from build123d import *

# Parameters (mm, degrees)
DODANIE_WYCI_GNI_CIE1_DEPTH = 15
SZKIC1_3_R                  = 6
DODANIE_WYCI_GNI_CIE2_DEPTH = 1
SZKIC1_4_R                  = 6
SZKIC1_4_R_2                = 5
DODANIE_WYCI_GNI_CIE3_DEPTH = 11
ZAOKR_GLENIE1_R             = 3
ZAOKR_GLENIE2_R             = 0.5
ZAOKR_GLENIE3_R             = 1


with BuildPart() as part:
    # Szkic1 → Dodanie-wyci_gni_cie1 (new body)
    with BuildSketch(Plane(origin=(0, 0, 0), x_dir=(1, 0, 0), z_dir=(0, 1, 0))):
        with BuildLine():
            Line((-26.353622573, 20), (26.353622573, 20))
            ThreePointArc((26.353622573, 20), (32.113981294, 17.613981294), (34.5, 11.853622573))
            Line((34.5, 11.853622573), (34.5, -11.853622573))
            ThreePointArc((34.5, -11.853622573), (32.113981294, -17.613981294), (26.353622573, -20))
            Line((26.353622573, -20), (-26.353622573, -20))
            ThreePointArc((-26.353622573, -20), (-32.113981294, -17.613981294), (-34.5, -11.853622573))
            Line((-34.5, -11.853622573), (-34.5, 11.853622573))
            ThreePointArc((-34.5, 11.853622573), (-32.113981294, 17.613981294), (-26.353622573, 20))
        make_face()
        with BuildLine():
            Line((-26.353622573, 19), (26.353622573, 19))
            ThreePointArc((26.353622573, 19), (31.406874513, 16.906874513), (33.5, 11.853622573))
            Line((33.5, 11.853622573), (33.5, -11.853622573))
            ThreePointArc((33.5, -11.853622573), (31.406874513, -16.906874513), (26.353622573, -19))
            Line((26.353622573, -19), (-26.353622573, -19))
            ThreePointArc((-26.353622573, -19), (-31.406874513, -16.906874513), (-33.5, -11.853622573))
            Line((-33.5, -11.853622573), (-33.5, 11.853622573))
            ThreePointArc((-33.5, 11.853622573), (-31.406874513, 16.906874513), (-26.353622573, 19))
        make_face(mode=Mode.SUBTRACT)
    extrude(amount=DODANIE_WYCI_GNI_CIE1_DEPTH)

    # Szkic1_3 → Dodanie-wyci_gni_cie2 (add)
    with BuildSketch(Plane(origin=(0, 0, 0), x_dir=(1, 0, 0), z_dir=(0, 1, 0))):
        with BuildLine():
            Line((-26.353622573, 19), (26.353622573, 19))
            ThreePointArc((26.353622573, 19), (31.406874513, 16.906874513), (33.5, 11.853622573))
            Line((33.5, 11.853622573), (33.5, -11.853622573))
            ThreePointArc((33.5, -11.853622573), (31.406874513, -16.906874513), (26.353622573, -19))
            Line((26.353622573, -19), (-26.353622573, -19))
            ThreePointArc((-26.353622573, -19), (-31.406874513, -16.906874513), (-33.5, -11.853622573))
            Line((-33.5, -11.853622573), (-33.5, 11.853622573))
            ThreePointArc((-33.5, 11.853622573), (-31.406874513, 16.906874513), (-26.353622573, 19))
        make_face()
        with Locations(Location((-22.5, 0, 0), (0, 0, 270))):
            Circle(SZKIC1_3_R, mode=Mode.SUBTRACT)
    extrude(amount=DODANIE_WYCI_GNI_CIE2_DEPTH)

    # Szkic1_4 → Dodanie-wyci_gni_cie3 (add)
    with BuildSketch(Plane(origin=(0, 0, 0), x_dir=(1, 0, 0), z_dir=(0, 1, 0))):
        with Locations(Location((-22.5, 0, 0), (0, 0, 270))):
            Circle(SZKIC1_4_R)
        with Locations(Location((-22.5, 0, 0), (0, 0, 270))):
            Circle(SZKIC1_4_R_2, mode=Mode.SUBTRACT)
    extrude(amount=DODANIE_WYCI_GNI_CIE3_DEPTH)

    # Zaokr_glenie1
    zaokr_glenie1_edges = [part.edges().sort_by_distance(p)[0] for p in [
        (32.113981294, 0, -17.613981294),
        (0, 0, -20),
        (-32.113981294, 0, -17.613981294),
        (-34.5, 0, 0),
        (-32.113981294, 0, 17.613981294),
        (0, 0, 20),
        (32.113981294, 0, 17.613981294),
        (34.5, 0, 0),
    ]]
    fillet(zaokr_glenie1_edges, radius=ZAOKR_GLENIE1_R)

    # Wyci_gni_cie po _cie_ce1: sweep along a path in Szkic2
    with BuildLine(Plane(origin=(0, 13, 0), x_dir=(1, 0, 0), z_dir=(0, 1, 0))) as wyci_gni_cie_po_cie_ce1_path:
        Line((-26.353622573, 20), (26.353622573, 20))
        ThreePointArc((26.353622573, 20), (32.113981294, 17.613981294), (34.5, 11.853622573))
        Line((34.5, 11.853622573), (34.5, -11.853622573))
        ThreePointArc((34.5, -11.853622573), (32.113981294, -17.613981294), (26.353622573, -20))
        Line((26.353622573, -20), (-26.353622573, -20))
        ThreePointArc((-26.353622573, -20), (-32.113981294, -17.613981294), (-34.5, -11.853622573))
        Line((-34.5, -11.853622573), (-34.5, 11.853622573))
        ThreePointArc((-34.5, 11.853622573), (-32.113981294, 17.613981294), (-26.353622573, 20))
    # Szkic3 → Wyci_gni_cie po _cie_ce1 (sweep)
    with BuildSketch(Plane(origin=(0, 0, 0), x_dir=(0, 0, -1), z_dir=(1, 0, 0))):
        with BuildLine():
            Line((20, 13), (20.5, 13))
            Line((20.5, 13), (20.5, 11.5))
            ThreePointArc((20.5, 11.5), (20.353553391, 11.146446609), (20, 11))
            Line((20, 11), (20, 13))
        make_face()
    sweep(path=wyci_gni_cie_po_cie_ce1_path.line)

    # Zaokr_glenie2
    zaokr_glenie2_edges = [part.edges().sort_by_distance(p)[0] for p in [
        (-22.5, 0, -5),
    ]]
    fillet(zaokr_glenie2_edges, radius=ZAOKR_GLENIE2_R)

    # Zaokr_glenie3
    zaokr_glenie3_edges = [part.edges().sort_by_distance(p)[0] for p in [
        (0, 1, -19),
        (-31.406874513, 1, 16.906874513),
        (31.406874513, 1, 16.906874513),
        (33.5, 1, 0),
        (31.406874513, 1, -16.906874513),
        (-31.406874513, 1, -16.906874513),
        (-33.5, 1, 0),
        (0, 1, 19),
    ]]
    fillet(zaokr_glenie3_edges, radius=ZAOKR_GLENIE3_R)


solid = part.part
Part model, mm, in its own coordinate system. A direction names the side the tool comes from. Round coordinates to 2 decimals unless told otherwise and drop trailing zeros. Write each loop counter-clockwise with the first axis right and the second up, starting at its lowest first coordinate (ties: lowest second). Pieces come first, ordered by that corner, then holes. Notation, with made-up numbers: M -27,71 L -3,71 A34 ccw -3,109 Z; hole C 59,17.25 d8. An arc over 180 degrees is marked long. Return JSON: item names as keys, results as strings. Group by question number.
(1) Pin check, flat tips, straight feed: pin 1 Ø13 at (x, z) = (-25.5, 2) entering from +Y; pin 2 Ø2.5 at (x, y) = (2.5, 6.5) entering from +Z; pin 3 Ø1 at (x, y) = (-20.5, 7.5) entering from -Z; pin 4 Ø12 at (x, z) = (-10, -10.5) entering from -Y. Stop position of each tip, or through.
(2) Saw through at D-D on y = 14.25. Write the cut outline in (x, z).
(3) Two-plate mould, pull along X, no slides. Class faces 5 (the face through (-32.18, 6.94, -17.55)), 6 (the face through (32.18, 6.94, 17.55)), 7 (the face through (0.2, 15, -19.4)), 8 (the face through (0, 8, -19)): +X half, -X half, draft (parallel to the pull), parting line (faces both ways), or undercut.
(4) Saw through at B-B on y = 5.75. Write the cut outline in (x, z).
(5) Drill centre lines: probe 1 along X at (y, z) = (5.75, 0); probe 2 along X at (y, z) = (12, 9.5); probe 3 along Z at (x, y) = (11.5, 9.5). Where is each one in solid material? Low to high.
(6) Which spindle directions (+Z, -Z, +X, -X, +Y, -Y) get a long thin tool onto all of the face, cutting with end or side? Do faces 1 (the face through (-31.462, 8.409, -16.851)), 2 (the face through (-34.5, 7, 0)), 3 (the face through (32.05, 6.94, -17.68)), 4 (the face through (-32.05, 13.99, 17.68)). Say none if no direction does.
Returned:
{
 "1": {"pin 1": "y = 11", "pin 2": "z = 20", "pin 3": "z = -20", "pin 4": "y = 0"},
 "2": {"outline": "M -34.5,-11.85 A8.15 ccw -26.35,-20 L 26.35,-20 A8.15 ccw 34.5,-11.85 L 34.5,11.85 A8.15 ccw 26.35,20 L -26.35,20 A8.15 ccw -34.5,11.85 Z; hole M -33.5,-11.85 A7.15 ccw -26.35,-19 L 26.35,-19 A7.15 ccw 33.5,-11.85 L 33.5,11.85 A7.15 ccw 26.35,19 L -26.35,19 A7.15 ccw -33.5,11.85 Z"},
 "3": {"face 5": "-X half", "face 6": "+X half", "face 7": "draft", "face 8": "undercut"},
 "4": {"outline": "M -34.5,-11.85 A8.15 ccw -26.35,-20 L 26.35,-20 A8.15 ccw 34.5,-11.85 L 34.5,11.85 A8.15 ccw 26.35,20 L -26.35,20 A8.15 ccw -34.5,11.85 Z; C -22.5,0 d12; hole M -33.5,-11.85 A7.15 ccw -26.35,-19 L 26.35,-19 A7.15 ccw 33.5,-11.85 L 33.5,11.85 A7.15 ccw 26.35,19 L -26.35,19 A7.15 ccw -33.5,11.85 Z; hole C -22.5,0 d10"},
 "5": {"probe 1": "-34.5 to -33.5, -28.5 to -27.5, -17.5 to -16.5, 33.5 to 34.5", "probe 2": "-35 to -33.5, 33.5 to 35", "probe 3": "-20 to -19, 19 to 20"},
 "6": {"face 1": "+Y", "face 2": "+Z, -Z, -X, -Y", "face 3": "-Z, +X, -Y", "face 4": "+Z, -X, +Y"}
}
